Can you work these out from the model? Positions are in its coordinate system, mm. A direction names the side the tool comes from. Coordinates: 2 decimals unless noted, no trailing zeros. Loops run counter-clockwise (first coordinate to the right, second up) from the corner with the lowest first, then second, coordinate; pieces in that order, holes last. Notation, with made-up numbers: (59.25, 0.25) -> (116.25, 0.25) arc R21 cw to (116.25, 24.25) -> close; hole circle Ø8 at (22.25, 68.5). An arc over 180 degrees is marked (long way). Use one line per item in the form item = value. Start each with the question number.
(1) Imagine slicing it at D-D (x = -109). List the corners of the cut face in (y, z) for me.
(2) Imagine slicing it at B-B (y = 45). List the corners of the cut face in (x, z) for me.
(3) I'm going to push flat-ended pins straight in: pin 1 (5 mm diameter, centred on x = -102.5, z = 5.5, fed in from +Y); pin 2 (1.5 mm diameter, centred on y = 46, z = 2, fed in from +X); pin 3 (4 mm diameter, centred on x = -31, z = 2, fed in from +Y). Where does each tip first touch, or does it pass through?
(4) On a 3-axis mill with a long thin cutter (end or side, diameter ignored), from which of +Z, -Z, +X, -X, +Y, -Y can I reach the whole of each face in a straight line? I mean faces 4 (the flat face through (-125, 15, 5)), 5 (the flat face through (0, 5, 5)), 6 (the flat face through (-43, 70, 5)), 7 (the flat face through (-82.09, 20.23, 4.93)), 8 (the flat face through (-8.7, 18.21, 4.93)). Say none if no direction works.
(5) Imagine slicing it at C-C (x = -35). List the corners of the cut face in (y, z) for me.
(6) Thinking about a two-plate mould opening in X: for faces 1 (the flat face through (-85.43, 34.32, 4.93)), 2 (the flat face through (-115, 7, 5)), 3 (the flat face through (-6.73, 37.26, 4.93)), which applies, released by +X, released by -X, zero draft, split by the parting line, or undercut?
(7) I need wall thicknesses on line 1 (Y direction, x = -35, z = 7.25); line 2 (X direction, y = 39, z = 4.25); line 3 (Y direction, x = -59.5, z = 6). Which ranges of each line are inside material? Lowest first, please. Write a range as [from, to].
(8) Imagine slicing it at A-A (z = 6). List the corners of the cut face in (x, y) for me.
```python
from build123d import *

# Parameters (mm, degrees)
CROQUIS1_R              = 12.5
CROQUIS1_R_2            = 7.5
SALIENTE_EXTRUIR1_DEPTH = 10


with BuildPart() as part:
    # Croquis1 → Saliente-Extruir1 (new body)
    with BuildSketch(Plane.XY):
        Polygon((0, 0), (-115, 0), (-115, 15), (-135, 15), (-135, 55), (-105, 55), (-105, 75), (-85, 95), (-55, 95), (-55, 70), (-30, 70), (3.419129876, 48.019059203), (-17.168499063, 26.198208287), (0, 10), align=None)
        with Locations((-55, 45)):
            Circle(CROQUIS1_R, mode=Mode.SUBTRACT)
        with Locations((-35, 15)):
            Circle(CROQUIS1_R_2, mode=Mode.SUBTRACT)
        Polygon((-105, 32.67766953), (-87.32233047, 15), (-76.715728753, 25.606601718), (-94.393398282, 43.284271247), align=None, mode=Mode.SUBTRACT)
    extrude(amount=SALIENTE_EXTRUIR1_DEPTH)


solid = part.part
```
Worked out:
q1.outline = (0, 0) -> (55, 0) -> (55, 10) -> (0, 10) -> close
q2.outline = (-135, 0) -> (-67.5, 0) -> (-67.5, 10) -> (-135, 10) -> close; (-42.5, 0) -> (0.57, 0) -> (0.57, 10) -> (-42.5, 10) -> close
q3.pin_1 = 80
q3.pin_2 = 2.22
q3.pin_3 = 70
q4.face_4 = +Z, -Z, -X, -Y
q4.face_5 = +Z, -Z, +X, -Y
q4.face_6 = +Z, -Z, +X, +Y
q4.face_7 = +Z, -Z
q4.face_8 = +Z, -Z, +X
q5.outline = (0, 0) -> (7.5, 0) -> (7.5, 10) -> (0, 10) -> close; (22.5, 0) -> (70, 0) -> (70, 10) -> (22.5, 10) -> close
q6.face_1 = undercut
q6.face_2 = released by -X
q6.face_3 = released by +X
q7.line_1 = [0, 7.5], [22.5, 70]
q7.line_2 = [-135, -98.68], [-90.11, -65.97], [-44.03, -5.09]
q7.line_3 = [0, 33.34], [56.66, 95]
q8.outline = (-135, 15) -> (-115, 15) -> (-115, 0) -> (0, 0) -> (0, 10) -> (-17.17, 26.2) -> (3.42, 48.02) -> (-30, 70) -> (-55, 70) -> (-55, 95) -> (-85, 95) -> (-105, 75) -> (-105, 55) -> (-135, 55) -> close; hole (-105, 32.68) -> (-87.32, 15) -> (-76.72, 25.61) -> (-94.39, 43.28) -> close; hole circle Ø25 at (-55, 45); hole circle Ø15 at (-35, 15)
